For this review, take the finished solid that the model builds, in its own axes (mm). A direction names the side the tool comes from. Coordinates: 2 decimals unless noted, no trailing zeros. Loops run counter-clockwise (first coordinate to the right, second up) from the corner with the lowest first, then second, coordinate; pieces in that order, holes last. Notation, with made-up numbers: (34.25, 45.25) -> (44.25, 45.25) arc R21 ccw to (44.25, 79.25) -> close; hole circle Ø7 at (-32, 39.25). An arc over 180 degrees is marked (long way). Answer in a Markdown table with one row per item.
from build123d import *

# Parameters (mm, degrees)
F0_W     = 10
F0_H     = 3
F1_DEPTH = 1
F2_DEPTH = 0.5
F3_R     = 0.2
F4_R     = 0.49999


# Not quite as in the source:
# - a fillet or chamfer is up to 0.001 mm smaller than in the source, because OpenCascade refuses the exact size


with BuildPart() as f1:
    # F0 (on Front) → F1 (new body)
    with BuildSketch(Plane.XZ):
        with Locations((-12.5, 0.0299999826)):
            Rectangle(F0_W, F0_H)
        Polygon((-6.1200000346, 15), (-7.5, 15), (-7.5, 1.5299999826), (-7.5, -1.4700000174), (-7.5, -15), (-6.1200000346, -15), (-6.1200000346, -12), (5.8799999654, -12), (5.8799999654, -15), (7.5, -15), (7.5, 15), (5.8799999654, 15), (5.8799999654, 12), (-6.1200000346, 12), align=None)
    extrude(amount=F1_DEPTH)

    # F0 (on Front) → F2 (cut)
    with BuildSketch(Plane.XZ):
        with Locations((-12.5, 0.0299999826)):
            Rectangle(F0_W, F0_H)
    extrude(amount=F2_DEPTH, mode=Mode.SUBTRACT)

    # F3
    f3_edges = [f1.edges().sort_by_distance(p)[0] for p in [
        (-12.5, -0.5, -1.47),
        (-12.5, -0.5, 1.53),
        (-12.5, -1, -1.47),
        (-12.5, -1, 1.53),
        (-17.5, -1, 0.03),
        (-17.5, -0.5, 0.03),
    ]]
    fillet(f3_edges, radius=F3_R)

    # F4 (radius 0.5 in the source; OpenCascade refuses exactly that, so slightly less here)
    f4_edges = [f1.edges().sort_by_distance(p)[0] for p in [
        (-0.12, -1, -12),
        (-0.12, -1, 12),
        (-0.12, 0, -12),
        (-0.12, 0, 12),
    ]]
    fillet(f4_edges, radius=F4_R)


solid = f1.part
Item 1: Take a section at A-A, the plane y = -0.2. State the section outline as (x, z) points, and give its area (3 significant figures).
Worked answers:
| item | result |
|---|---|
| outline | (-7.5, -15) -> (-6.12, -15) -> (-6.12, -11.9) -> (5.88, -11.9) -> (5.88, -15) -> (7.5, -15) -> (7.5, 15) -> (5.88, 15) -> (5.88, 11.9) -> (-6.12, 11.9) -> (-6.12, 15) -> (-7.5, 15) -> close |
| area | 376 mm² |
Item 2: Take a section at B-B, the plane x = -9.75. State the section outline as (y, z) points, and give its area (3 significant figures).
Worked answers:
| item | result |
|---|---|
| outline | (-1, -1.27) arc R0.2 ccw to (-0.8, -1.47) -> (-0.7, -1.47) arc R0.2 ccw to (-0.5, -1.27) -> (-0.5, 1.33) arc R0.2 ccw to (-0.7, 1.53) -> (-0.8, 1.53) arc R0.2 ccw to (-1, 1.33) -> close |
| area | 1.47 mm² |
Item 3: The part is to be moulded in two halves that separate along X. For faces 3 (the flat face through (5.88, -0.5, -13.6)), 4 (the flat face through (-7.5, -0.3, -0.2)), 5 (the flat face through (-6.12, -0.5, 13.6)), 6 (the flat face through (6.7, -0.5, 15)), say which applies: +X half, -X half, draft (parallel to the pull), parting line (faces both ways), or undercut.
Worked answers:
| item | result |
|---|---|
| face 3 | undercut |
| face 4 | -X half |
| face 5 | undercut |
| face 6 | draft |
Item 4: Insertion check: pin 1 (1.3 mm diameter, centred on x = -13, z = 0, fed in from +Y); pin 2 (0.5 mm diameter, centred on y = -0.5, z = -3, fed in from -X). Each pin has a flat end and moves straight along its axis. Give the tip position at first contact, or say it passes through.
Worked answers:
| item | result |
|---|---|
| pin 1 | y = -0.5 |
| pin 2 | x = -7.5 |
Item 5: Take a section at C-C, the plane z = 6. State the section outline as (x, y) points.
Worked answers:
| item | result |
|---|---|
| outline | (-7.5, -1) -> (7.5, -1) -> (7.5, 0) -> (-7.5, 0) -> close |
Item 6: For L1, parallel to X at y = -0.9, z = -12.5; L2, parallel to X at y = -0.9, z = 2.5; L3, parallel to Z at x = 5.25, y = -0.5, list the stretches that pass through material, from the lowest coordinate up.
Worked answers:
| item | result |
|---|---|
| L1 | -7.5 to -6.12, 5.88 to 7.5 |
| L2 | -7.5 to 7.5 |
| L3 | -12 to 12 |
Item 7: For faces 1 (the flat face through (7.5, -0.5, -0.2)), 2 (the flat face through (-12, -0.5, 0)), list the 3-axis set-ups (+Z, -Z, +X, -X, +Y, -Y) from which the entire face can be reached by the end or side of a thin tool; tool diameter is ignored.
Worked answers:
| item | result |
|---|---|
| face 1 | +Z, -Z, +X, +Y, -Y |
| face 2 | +Z, -Z, -X, +Y |
